Here's how the part is built. I have some questions about the finished solid (model axes, mm). A direction names the side the tool comes from. Give positions to 0.01 mm unless a question says otherwise; leave off trailing zeros. Loops run counter-clockwise (first coordinate to the right, second up) from the corner with the lowest first, then second, coordinate; pieces in that order, holes last. Notation, with made-up numbers: M -1.5,70.5 L 23.5,70.5 A29 cw 23.5,100.5 Z; hole C 1,25.25 d8. An arc over 180 degrees is marked long. Answer as CSV lines item,"result". Start each with the question number.
Item 1: If we mould it in two halves opening along Y, with no side actions, what happens to faces 1 (the flat face through (27, 9.525, 15)), 2 (the cylindrical face through (11.115, -10.611, 13.952)), 3 (the flat face through (0, -13, 15.24))? For each: released by +Y, released by -Y, zero draft, split by the parting line, or undercut.
Item 2: I want a section at A-A on z = 0. List the corners of the cut face in (x, y) for me, plus the area to 3 significant figures.
Item 3: If I drill on line 1 along X through (y, z) = (17.25, 0); line 2 along Y through (x, z) = (-12.5, -4); line 3 along Y through (x, z) = (-18.5, 14) (3 decimals), over which ranges is the centre line in solid material (lowest first)? Write a range as from..to.
Item 4: For faces 4 (the flat face through (9.97, -49, 15)), 5 (the flat face through (-28, 9.525, 15)), 6 (the flat face through (-33.655, 0, 19)), which set-ups out of +Z, -Z, +X, -X, +Y, -Y let a thin tool reach every point of the face, with its end or its side?
Item 5: I want a section at D-D on z = 7. List the corners of the cut face in (x, y) for me.
Item 6: Will these pins go through, and if not, where does the flat tip stop? P1, Ø1.5, axis at y = -18, z = 10, coming from the -X side; P2, Ø5, axis at x = -16, y = -1, coming from the +Z side; P3, Ø6, axis at x = 18, y = 1, coming from the -Z side.
from build123d import *

# Parameters (mm, degrees)
F1_DEPTH       = 25.4
F1_DEPTH_BACK  = 25.4
F2_W           = 25.4
F2_H           = 40.9454388922
F3_DEPTH       = 25.4
F3_DEPTH_BACK  = 25.4
F4_W           = 19.939
F4_H           = 2.54
F5_DEPTH       = 25.4
F5_DEPTH_BACK  = 25.4
F7_DEPTH       = 9.525
F7_DEPTH_BACK  = 9.525
F8_R           = 3.81
F10_DEPTH      = 9.9695
F10_DEPTH_BACK = 9.9695
F11_SIZE       = 1.27
F12_SIZE       = 1.27


with BuildPart() as f1:
    # F0 (on Front) → F1 (new body, two sides)
    with BuildSketch(Plane.XZ) as f1_sk:
        with BuildLine():
            Line((8.09625, -9.7847195125), (9.411890625, -11.3747364332))
            ThreePointArc((9.411890625, -11.3747364332), (0, 14.76375), (-9.411890625, -11.3747364332))
            Line((-9.411890625, -11.3747364332), (-8.09625, -9.7847195125))
            ThreePointArc((-8.09625, -9.7847195125), (0, 12.7), (8.09625, -9.7847195125))
        make_face()
    extrude(amount=F1_DEPTH)
    extrude(f1_sk.sketch, amount=-F1_DEPTH_BACK)

    # F2 (on Right) → F3 (cut, two sides)
    with BuildSketch(Plane.YZ) as f3_sk:
        with Locations((0, 1.1786520481)):
            Rectangle(F2_W, F2_H)
    extrude(amount=-F3_DEPTH, mode=Mode.SUBTRACT)
    extrude(f3_sk.sketch, amount=F3_DEPTH_BACK, mode=Mode.SUBTRACT)

    # F4 (on Front) → F5 (join, two sides)
    with BuildSketch(Plane.XZ) as f5_sk:
        with Locations((0, 13.97)):
            Rectangle(F4_W, F4_H)
    extrude(amount=F5_DEPTH)
    extrude(f5_sk.sketch, amount=-F5_DEPTH_BACK)

    # F6 (on Front) → F7 (join, two sides)
    with BuildSketch(Plane.XZ) as f7_sk:
        with BuildLine():
            Line((-33.655, 12.7), (0, 12.7))
            Line((0, 12.7), (0, 15.24))
            Line((0, 15.24), (-33.02, 15.24))
            ThreePointArc((-33.02, 15.24), (-33.4690128061, 15.4259871939), (-33.655, 15.875))
            Line((-33.655, 15.875), (-33.655, 22.225))
            Line((-33.655, 22.225), (-33.3598416866, 22.225))
            ThreePointArc((-33.3598416866, 22.225), (-33.0602119039, 22.3001366298), (-32.8314897497, 22.5077653754))
            Line((-32.8314897497, 22.5077653754), (-32.385, 23.1775))
            Line((-32.385, 23.1775), (-32.385, 24.13))
            Line((-32.385, 24.13), (-35.814, 24.13))
            Line((-35.814, 24.13), (-35.814, 22.225))
            Line((-35.814, 22.225), (-35.814, 13.335))
            ThreePointArc((-35.814, 13.335), (-35.6280128061, 12.8859871939), (-35.179, 12.7))
            Line((-35.179, 12.7), (-33.655, 12.7))
        make_face()
        with BuildLine():
            Line((0, 15.24), (0, 12.7))
            Line((0, 12.7), (33.655, 12.7))
            Line((33.655, 12.7), (35.179, 12.7))
            ThreePointArc((35.179, 12.7), (35.6280128061, 12.8859871939), (35.814, 13.335))
            Line((35.814, 13.335), (35.814, 22.225))
            Line((35.814, 22.225), (35.814, 24.13))
            Line((35.814, 24.13), (32.385, 24.13))
            Line((32.385, 24.13), (32.385, 23.1775))
            Line((32.385, 23.1775), (32.8314897497, 22.5077653754))
            ThreePointArc((32.8314897497, 22.5077653754), (33.0602119039, 22.3001366298), (33.3598416866, 22.225))
            Line((33.3598416866, 22.225), (33.655, 22.225))
            Line((33.655, 22.225), (33.655, 15.875))
            ThreePointArc((33.655, 15.875), (33.4690128061, 15.4259871939), (33.02, 15.24))
            Line((33.02, 15.24), (0, 15.24))
        make_face()
    extrude(amount=F7_DEPTH)
    extrude(f7_sk.sketch, amount=-F7_DEPTH_BACK)

    # F8
    f8_edges = [f1.edges().sort_by_distance(p)[0] for p in [
        (-9.9695, 9.525, 13.97),
        (9.9695, 9.525, 13.97),
        (9.9695, -9.525, 13.97),
        (-9.9695, -9.525, 13.97),
    ]]
    fillet(f8_edges, radius=F8_R)

    # F9 (on Right) → F10 (join, two sides)
    with BuildSketch(Plane.YZ) as f10_sk:
        with BuildLine():
            Line((-72.39, 12.7), (0, 12.7))
            Line((0, 12.7), (0, 15.24))
            Line((0, 15.24), (-71.755, 15.24))
            ThreePointArc((-71.755, 15.24), (-72.2040128061, 15.4259871939), (-72.39, 15.875))
            Line((-72.39, 15.875), (-72.39, 22.225))
            Line((-72.39, 22.225), (-69.85, 22.225))
            Line((-69.85, 22.225), (-68.58, 23.1775))
            Line((-68.58, 23.1775), (-68.58, 24.13))
            Line((-68.58, 24.13), (-72.39, 24.13))
            Line((-72.39, 24.13), (-74.93, 24.13))
            Line((-74.93, 24.13), (-74.93, 13.335))
            ThreePointArc((-74.93, 13.335), (-74.7440128061, 12.8859871939), (-74.295, 12.7))
            Line((-74.295, 12.7), (-72.39, 12.7))
        make_face()
    extrude(amount=F10_DEPTH)
    extrude(f10_sk.sketch, amount=-F10_DEPTH_BACK)

    # F11
    f11_edges = [f1.edges().sort_by_distance(p)[0] for p in [
        (-9.9695, 25.4, 13.97),
        (9.9695, 25.4, 13.97),
    ]]
    chamfer(f11_edges, length=F11_SIZE)

    # F12
    f12_edges = [f1.edges().sort_by_distance(p)[0] for p in [
        (0, -74.93, 24.13),
        (-35.814, 0, 24.13),
        (35.814, 0, 24.13),
    ]]
    chamfer(f12_edges, length=F12_SIZE)


solid = f1.part
Result:
1,face 1,"released by +Y"
1,face 2,"released by -Y"
1,face 3,"zero draft"
2,outline,"M -14.76,-25.4 L -12.7,-25.4 L -12.7,-12.7 L -14.76,-12.7 Z; M -14.76,12.7 L -12.7,12.7 L -12.7,25.4 L -14.76,25.4 Z; M 12.7,-25.4 L 14.76,-25.4 L 14.76,-12.7 L 12.7,-12.7 Z; M 12.7,12.7 L 14.76,12.7 L 14.76,25.4 L 12.7,25.4 Z"
2,area,"105 mm^2"
3,line 1,"-14.76..-12.7, 12.7..14.76"
3,line 2,"-25.4..-12.7, 12.7..25.4"
3,line 3,"-9.525..9.525"
4,face 4,"+Z, +X, -Y"
4,face 5,"+Z, -Z, -X, +Y"
4,face 6,"+Y, -Y"
5,outline,"M -13,-25.4 L -10.6,-25.4 L -10.6,-12.7 L -13,-12.7 Z; M -13,12.7 L -10.6,12.7 L -10.6,25.4 L -13,25.4 Z; M 10.6,-25.4 L 13,-25.4 L 13,-12.7 L 10.6,-12.7 Z; M 10.6,12.7 L 13,12.7 L 13,25.4 L 10.6,25.4 Z"
6,P1,"x = -11.51"
6,P2,"z = 15.24"
6,P3,"z = 12.7"
